Build history of the part. All positions in model axes, mm. Face numbers are marked on the shaded views. A direction names the side the tool comes from. Give positions to 0.01 mm unless a question says otherwise; leave off trailing zeros. Loops run counter-clockwise (first coordinate to the right, second up) from the corner with the lowest first, then second, coordinate; pieces in that order, holes last. Notation, with made-up numbers: M -24,-33 L 2,-33 A21 ccw 2,-25 Z; hole C 51,53 d1. An arc over 180 degrees is marked long. Answer in a Markdown table with one row per item. Add a question column.
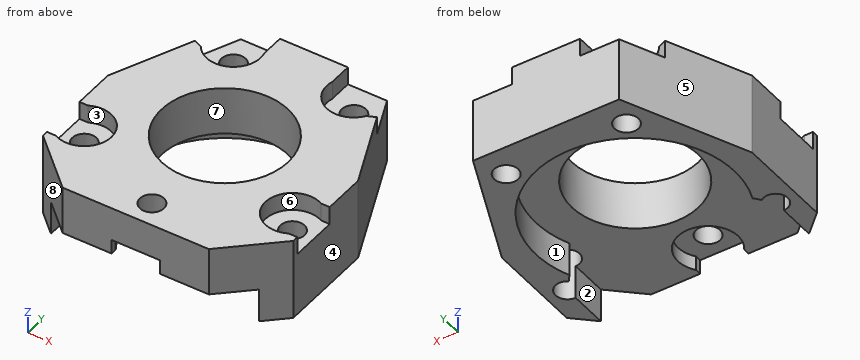
Autodesk Inventor part; units mm, degrees
ref_plane "Work Plane2" through (-10.3994, -22, -2.8) normal (0, 0, 1) x (1, 0, 0)
ref_plane "YZ Plane" through (0, 0, 0) normal (1, 0, 0) x (0, 1, 0)
ref_plane "XZ Plane" through (0, 0, 0) normal (0, 1, 0) x (-1, 0, 0)
ref_plane "Work Plane1" through (0, 0, 0) normal (0, 0, 1) x (1, 0, 0)
sketch "Sketch1" plane through (0, 0, 0) normal (0, 0, 1) x (1, 0, 0)
  line L0 (-6.075, -22) -> (6.075, -22)
  line L1 (-6.075, -22) -> (-10.3994, -18)
  line L2 (-10.3994, -18) -> (-10.3994, -10)
  line L3 (-10.3994, -10) -> (-6.075, 0)
  line L4 (6.075, 0) -> (-6.075, 0)
  line L5 (6.075, 0) -> (10.3994, -10)
  line L6 (10.3994, -10) -> (10.3994, -18)
  line L7 (10.3994, -18) -> (6.075, -22)
  circle A0 centre (0, -11) radius 3.4
  circle A1 centre (0, -20) radius 1
  circle A2 centre (8.6494, -15.5) radius 1
  circle A3 centre (-8.6494, -15.5) radius 1
  circle A4 centre (0, -20) radius 2.5
  line L8 (-2, -21.5) -> (-2, -22)
  line L9 (2, -21.5) -> (2, -22)
  line L10 (0, -20) -> (0, -22) construction
  circle A5 centre (0, -11) radius 5.25
  line L11 (0, 4.5) -> (0, -27)
  circle A6 centre (-5, -2.5) radius 1
  circle A7 centre (5, -2.5) radius 1
  point P0 (0, 0)
  dimension "d0" = 5
  dimension "d1" = 4
  dimension "d2" = 10.5
extrude "ext_main" add sketch "Sketch1" along normal blind 4 contours L1 L2 L3 L4 L11 A5 A4 L8 L0 | L8 A4 L0 | A4 L11 A1 L0 | L11 A1 A4 L0 | L11 A5 L4 L5 L6 L7 L0 L9 A4 | A4 L9 L0
sketch "Sketch2" plane through (0, 0, 0) normal (0, 0, -1) x (-1, 0, 0)
  circle A0 centre (0, -20) radius 2.5
  line L0 (-2, -21.5) -> (-2, -22)
  line L1 (2, -21.5) -> (2, -22)
  line L2 (-2, -22) -> (2, -22)
extrude "ext_cut_gearhousing" cut sketch "Sketch2" against normal blind 1.2
sketch "Sketch3" plane through (0, 0, 0) normal (0, 0, 1) x (1, 0, 0)
  line L0 (-10.3994, -18) -> (-10.3994, -10)
  line L1 (-6.075, -22) -> (-10.3994, -18)
  line L2 (-6.075, -22) -> (6.075, -22)
  line L3 (10.3994, -18) -> (6.075, -22)
  line L4 (10.3994, -10) -> (10.3994, -18)
  line L5 (6.075, 0) -> (10.3994, -10)
  line L6 (6.075, 0) -> (-6.075, 0)
  line L7 (-10.3994, -10) -> (-6.075, 0)
  circle A0 centre (-8.6494, -15.5) radius 1
  circle A1 centre (8.6494, -15.5) radius 1
  circle A2 centre (0, -20) radius 1
  circle A3 centre (0, -11) radius 3.4
  circle A4 centre (0, -20) radius 8 construction
  circle A5 centre (5.075, -11) radius 1
  circle A6 centre (-5.075, -11) radius 1
  circle A7 centre (-5.075, -11) radius 3 construction
  circle A8 centre (5.075, -11) radius 3 construction
  line L8 (-8.6494, -16.5) -> (-8.6494, -19.6187)
  line L9 (-5.075, -11) -> (-8.6494, -15.5) construction
  line L10 (5.075, -11) -> (8.6494, -15.5) construction
  line L11 (8.6494, -15.5) -> (8.6494, -19.6187) construction
  line L12 (8.6494, -16.5) -> (8.6494, -19.6187)
  arc A9 (-8.0274, -14.717) -> (-8.6494, -16.5) centre (-8.6494, -15.5) ccw
  arc A10 (8.6494, -16.5) -> (8.0274, -14.717) centre (8.6494, -15.5) ccw
  line L13 (-8.6494, -19.6187) -> (-10.3994, -18)
  line L14 (10.3994, -18) -> (8.6494, -19.6187)
  circle A11 centre (0, -11) radius 8.25 construction
  line L15 (-7.6085, -14.1895) -> (-8.0274, -14.717)
  line L16 (8.0274, -14.717) -> (7.6085, -14.1895)
  circle A12 centre (-5, -2.5) radius 1
  circle A13 centre (5, -2.5) radius 1
  arc A14 (7.6085, -14.1895) -> (-7.6085, -14.1895) centre (0, -11) ccw
  point P0 (-6.9409, -13.3491)
  point P1 (5.075, -8)
  point P2 (-5.075, -8)
  point P3 (6.9409, -13.3491)
  dimension "d7" = 16
  dimension "d8" = 6
  dimension "d20" = 16.5
ref_plane "Work Plane2" through (-10.3994, -22, -2.8) normal (0, 0, 1) x (1, 0, 0)
extrude "ext_base" add sketch "Sketch3" against normal up to surface (2.8 mm away) contours L0 L7 L6 L5 L4 L3 L12 A1 L16 A14 L15 A0 L8 L1
sketch "Sketch4" plane through (0, 0, 4) normal (0, 0, 1) x (1, 0, 0)
  circle A0 centre (8.6494, -15.5) radius 1
  circle A1 centre (-8.6494, -15.5) radius 1
  line L0 (10.3994, -18) -> (10.3994, -10)
  line L1 (-10.3994, -10) -> (-10.3994, -18)
  circle A2 centre (-8.6494, -15.5) radius 2.25
  circle A3 centre (8.6494, -15.5) radius 2.25
  line L2 (-9.6802, -13.5) -> (-10.3994, -13.5)
  line L3 (-9.6802, -17.5) -> (-10.3994, -17.5)
  line L4 (-8.6494, -15.5) -> (-10.3994, -15.5) construction
  line L5 (8.6494, -15.5) -> (10.3994, -15.5)
  line L6 (9.6802, -13.5) -> (10.3994, -13.5)
  line L7 (9.6802, -17.5) -> (10.3994, -17.5)
  circle A4 centre (-5, -2.5) radius 1
  circle A5 centre (5, -2.5) radius 1
  line L8 (10.3994, -10) -> (6.075, 0)
  line L9 (6.075, 0) -> (-6.075, 0)
  line L10 (-6.075, 0) -> (-10.3994, -10)
  circle A6 centre (-5, -2.5) radius 2.25
  circle A7 centre (5, -2.5) radius 2.25
  line L11 (-2.825, -1.9239) -> (-2.825, 0)
  line L12 (-6.8699, -3.7514) -> (-7.5669, -3.45)
  line L13 (0, 4.4) -> (0, -26.4)
  line L14 (2.825, -1.9239) -> (2.825, 0)
  line L15 (6.8699, -3.7514) -> (7.5669, -3.45)
  point P0 (0, 0)
  dimension "d11" = 4.5
  dimension "d12" = 4
  dimension "d13" = 4
  dimension "d18" = 3.25
  dimension "d19" = 3.45
extrude "ext_cut_screwheads" cut sketch "Sketch4" against normal blind 1.5 contours L0 A3 | L2 A2 L1 | L11 A6 L10 L9 | L15 A7 L8 | L0 L7 A3 | A3 L6 L0 | A7 L8 | L8 A7 | A7 L14 L9 L8 | A6 L10 | L10 A6 | A6 L12 L10 | A2 L1 | A2 L3 L1 | A4 | A5 picked at (10.1112, -14.8737) picked at (-10.1494, -15.5)
equation "\"d11\" = screw_m2_head_maxsize"
properties part number "linact_thumb_front"
(1) Wall check: line 1 (X direction, y = -11, z = -2); line 2 (X direction, y = -15.5, z = -0.6); line 3 (Y direction, x = 0, z = 0.6). Give the ranges that are in metal, low to high.
(2) Slice it at D-D, the plane z = -2. Give the cut face in (x, y) (1 decimal), then the cut area to 3 significant figures.
(3) Pin check, flat tips, straight feed: pin 1 (3.5 mm diameter, centred on x = 8.65, y = -15.5, fed in from +Z); pin 2 (5 mm diameter, centred on x = 5, y = -2, fed in from +Z); pin 3 (0.6 mm diameter, centred on y = -21.5, z = 1, fed in from -X); pin 4 (1.5 mm diameter, centred on y = -2.5, z = 2.5, fed in from -X). Stop position of each tip, or through.
(4) Slice it at C-C, the plane y = -15.5. Give the cut face in (x, z), then the cut area to 3 significant figures.
(5) Slice it at B-B, the plane x = 0.75. Give the cut face in (y, z), then the cut area to 3 significant figures.
(6) Tool access for the marked faces 1, 2, 3 and 4: list every direction of +Z, -Z, +X, -X, +Y, -Y with a clear straight run to the whole face (end or side of a thin tool).
(7) Slice it at A-A, the plane z = 0.5. Give the cut face in (x, y) (3 decimals).
(8) Pull direction Y, two halves, no side cores. Call the marked faces 5, 6, 7 and 8: +Y half, -Y half, draft (parallel to the pull), parting line (faces both ways), or undercut.
Solution:
| question | item | result |
|---|---|---|
| 1 | line 1 | -10.4 to -8.25, 8.25 to 10.4 |
| 1 | line 2 | -10.4 to -9.65, 9.65 to 10.4 |
| 1 | line 3 | -17.5 to -16.25, -5.75 to 0 |
| 2 | outline | M -10.4,-18 L -8.6,-19.6 L -8.6,-16.5 A1 cw long -8,-14.7 L -7.6,-14.2 A8.2 cw long 7.6,-14.2 L 8,-14.7 A1 cw long 8.6,-16.5 L 8.6,-19.6 L 10.4,-18 L 10.4,-10 L 6.1,0 L -6.1,0 L -10.4,-10 Z; hole C -5,-2.5 d2; hole C 5,-2.5 d2 |
| 2 | area | 101 mm^2 |
| 3 | pin 1 | z = 2.5 |
| 3 | pin 2 | z = 4 |
| 3 | pin 3 | x = -6.94 |
| 3 | pin 4 | x = -7.48 |
| 4 | outline | M -10.4,-2.8 L -9.65,-2.8 L -9.65,2.5 L -10.4,2.5 Z; M -7.65,0 L -2.7,0 L -2.7,4 L -6.4,4 L -6.4,2.5 L -7.65,2.5 Z; M 2.7,0 L 7.65,0 L 7.65,2.5 L 6.4,2.5 L 6.4,4 L 2.7,4 Z; M 9.65,-2.8 L 10.4,-2.8 L 10.4,2.5 L 9.65,2.5 Z |
| 4 | area | 43.8 mm^2 |
| 5 | outline | M -22,1.2 L -20.66,1.2 L -20.66,4 L -22,4 Z; M -19.34,1.2 L -17.62,1.2 L -17.62,0 L -16.2,0 L -16.2,4 L -19.34,4 Z; M -5.8,0 L -2.78,0 L -2.78,-2.8 L 0,-2.8 L 0,4 L -5.8,4 Z |
| 5 | area | 45.3 mm^2 |
| 6 | face 1 | -Z |
| 6 | face 2 | -Z, -Y |
| 6 | face 3 | +Z |
| 6 | face 4 | +Z, -Z, +X, +Y, -Y |
| 7 | outline | M -10.399,-18 L -6.075,-22 L -2,-22 L -2,-21.5 A2.5 cw long 2,-21.5 L 2,-22 L 6.075,-22 L 10.399,-18 L 10.399,-10 L 6.075,0 L -6.075,0 L -10.399,-10 Z; hole C -8.649,-15.5 d2; hole C -5,-2.5 d2; hole C 0,-11 d10.5; hole C 5,-2.5 d2; hole C 8.649,-15.5 d2 |
| 8 | face 5 | +Y half |
| 8 | face 6 | undercut |
| 8 | face 7 | undercut |
| 8 | face 8 | -Y half |
